```python
from build123d import *

# Parameters (mm, degrees)
EXTRUDE_1_DEPTH   = 5.08
EXTRUDE_1_2_DEPTH = 5.08
EXTRUDE_2_DEPTH   = 16
EXTRUDE_3_DEPTH   = 2.54
EXTRUDE_START     = 12.7
EXTRUDE_4_DEPTH   = 2.54
CHAMFER_1_SIZE    = 0.15


with BuildPart() as part:
    # Sketch 1 → Extrude 1 (new body)
    with BuildSketch(Plane(origin=(0, 0, 0), x_dir=(1, 0, 0), z_dir=(0, 1, 0))):
        Polygon((-1.59, -0.22), (-1.59, 0.22), (-1.49, 0.32), (-1.05, 0.32), (-0.95, 0.22), (-0.95, -0.22), (-1.05, -0.32), (-1.49, -0.32), align=None)
    extrude(amount=-EXTRUDE_1_DEPTH)



with BuildPart() as body_2:
    # Sketch 1 → Extrude 1 2 (new body)
    with BuildSketch(Plane(origin=(0, 0, 0), x_dir=(1, 0, 0), z_dir=(0, 1, 0))):
        Polygon((0.95, -0.22), (0.95, 0.22), (1.05, 0.32), (1.49, 0.32), (1.59, 0.22), (1.59, -0.22), (1.49, -0.32), (1.05, -0.32), align=None)
    extrude(amount=-EXTRUDE_1_2_DEPTH)


with BuildPart() as part_1:
    add(part.part)

    add(body_2.part)  # Extrude 2 merges body 2
    # Sketch 1_3 → Extrude 2 (add)
    with BuildSketch(Plane(origin=(0, 0, 0), x_dir=(1, 0, 0), z_dir=(0, 1, 0))):
        Polygon((-1.59, -0.22), (-1.59, 0.22), (-1.49, 0.32), (-1.05, 0.32), (-0.95, 0.22), (-0.95, -0.22), (-1.05, -0.32), (-1.49, -0.32), align=None)
        Polygon((0.95, -0.22), (0.95, 0.22), (1.05, 0.32), (1.49, 0.32), (1.59, 0.22), (1.59, -0.22), (1.49, -0.32), (1.05, -0.32), align=None)
    extrude(amount=EXTRUDE_2_DEPTH)

    # Sketch 1_4 → Extrude 3 (add)
    with BuildSketch(Plane(origin=(0, 0, 0), x_dir=(1, 0, 0), z_dir=(0, 1, 0))):
        Polygon((-2.54, 1.07), (-2.54, -1.07), (-2.34, -1.27), (-0.2, -1.27), (0, -1.07), (0, 1.07), (-0.2, 1.27), (-2.34, 1.27), align=None)
        Polygon((-1.59, -0.22), (-1.49, -0.32), (-1.05, -0.32), (-0.95, -0.22), (-0.95, 0.22), (-1.05, 0.32), (-1.49, 0.32), (-1.59, 0.22), align=None, mode=Mode.SUBTRACT)
        Polygon((0, 1.07), (0, -1.07), (0.2, -1.27), (2.34, -1.27), (2.54, -1.07), (2.54, 1.07), (2.34, 1.27), (0.2, 1.27), align=None)
        Polygon((0.95, -0.22), (1.05, -0.32), (1.49, -0.32), (1.59, -0.22), (1.59, 0.22), (1.49, 0.32), (1.05, 0.32), (0.95, 0.22), align=None, mode=Mode.SUBTRACT)
    extrude(amount=EXTRUDE_3_DEPTH)

    # Sketch 1_5 → Extrude 4 (add)
    with BuildSketch(Plane(origin=(0, 0, 0), x_dir=(1, 0, 0), z_dir=(0, 1, 0)).offset(EXTRUDE_START)):
        Polygon((-2.34, 1.27), (-0.2, 1.27), (0, 1.07), (0.2, 1.27), (2.34, 1.27), (2.54, 1.07), (2.54, -1.07), (2.34, -1.27), (0.2, -1.27), (0, -1.07), (-0.2, -1.27), (-2.34, -1.27), (-2.54, -1.07), (-2.54, 1.07), align=None)
    extrude(amount=-EXTRUDE_4_DEPTH)

    # Chamfer 1
    chamfer_1_edges = [part_1.edges().sort_by_distance(p)[0] for p in [
        (-1.27, -5.08, 0.32),
        (1.59, -5.08, 0),
        (1.54, -5.08, 0.27),
        (1.27, -5.08, 0.32),
        (1, -5.08, 0.27),
        (0.95, 16, 0),
        (1, 16, -0.27),
        (1.27, 16, -0.32),
        (1.54, 16, -0.27),
        (0.95, -5.08, 0),
        (1, -5.08, -0.27),
        (1.27, -5.08, -0.32),
        (1.54, -5.08, -0.27),
        (1, 16, 0.27),
        (1.27, 16, 0.32),
        (1.54, 16, 0.27),
        (1.59, 16, 0),
        (-1, -5.08, 0.27),
        (-0.95, -5.08, 0),
        (-1, -5.08, -0.27),
        (-1.59, 16, 0),
        (-1, 16, -0.27),
        (-1.27, 16, -0.32),
        (-1.54, 16, -0.27),
        (-1.27, -5.08, -0.32),
        (-1.54, 16, 0.27),
        (-1.27, 16, 0.32),
        (-1, 16, 0.27),
        (-0.95, 16, 0),
        (-1.54, -5.08, -0.27),
        (-1.59, -5.08, 0),
        (-1.54, -5.08, 0.27),
    ]]
    chamfer(chamfer_1_edges, length=CHAMFER_1_SIZE)


solid = part_1.part
```
Source: CAD feature listing. Evaluate the final solid. Frame: model axes, mm. Give positions to 0.01 mm unless a question says otherwise; leave off trailing zeros. Loops run counter-clockwise (first coordinate to the right, second up) from the corner with the lowest first, then second, coordinate; pieces in that order, holes last. Notation, with made-up numbers: (66.25, -21) -> (102.25, -21) arc R24 ccw to (102.25, 15) -> close; hole circle Ø7 at (48, -30). An arc over 180 degrees is marked (long way). Put each result on its own line as item: value. Start each with the question number.
1) Contact query for flat-ended pins moving along their axis: P1, Ø1, axis at x = 0.5, z = -0.5, coming from the +Y side; P2, Ø0.5, axis at x = -1.5, y = 8, coming from the +Z side; P3, Ø0.5, axis at x = -1, y = -2.5, coming from the -Z side. Output: stop coordinate, or through.
2) Cut plane B-B (z = -0.7). Return loops of the section in (x, y), then the cut area to 3 significant figures.
3) Material intervals for probe 1 along Y at (x, z) = (1.65, 0.4); probe 2 along X at (y, z) = (-1.75, -0.15), sorted ascending.
4) Draft query along Y for faces 1 (the face through (0, 10.16, 0)), 2 (the face through (0, 2.54, 0)), 3 (the face through (2.54, 1, 0)), 4 (the face through (0, 12.7, 0)). Return one class per face: released by +Y, released by -Y, zero draft, split by the parting line, or undercut.
5) Cut plane C-C (x = 0.55). Return loops of the section in (y, z), then the cut area to 3 significant figures.
6) Cut plane A-A (y = 5.5). Return loops of the section in (x, z).
Results are:
1. P1: stops at y = 12.7
1. P2: stops at z = 0.32
1. P3: stops at z = -0.32
2. outline: (-2.54, 0) -> (2.54, 0) -> (2.54, 2.54) -> (-2.54, 2.54) -> close; (-2.54, 10.16) -> (2.54, 10.16) -> (2.54, 12.7) -> (-2.54, 12.7) -> close
2. area: 25.8 mm2
3. probe 1: y = 0 to 2.54, 10.16 to 12.7
3. probe 2: x = -1.59 to -0.95, 0.95 to 1.59
4. face 1: undercut
4. face 2: undercut
4. face 3: zero draft
4. face 4: released by +Y
5. outline: (0, -1.27) -> (2.54, -1.27) -> (2.54, 1.27) -> (0, 1.27) -> close; (10.16, -1.27) -> (12.7, -1.27) -> (12.7, 1.27) -> (10.16, 1.27) -> close
5. area: 12.9 mm2
6. outline: (-1.59, -0.22) -> (-1.49, -0.32) -> (-1.05, -0.32) -> (-0.95, -0.22) -> (-0.95, 0.22) -> (-1.05, 0.32) -> (-1.49, 0.32) -> (-1.59, 0.22) -> close; (0.95, -0.22) -> (1.05, -0.32) -> (1.49, -0.32) -> (1.59, -0.22) -> (1.59, 0.22) -> (1.49, 0.32) -> (1.05, 0.32) -> (0.95, 0.22) -> close
